CAD build for the part. Positions are in the model's coordinates, mm. Face numbers are marked on the shaded views. A direction names the side the tool comes from. Coordinates: 2 decimals unless noted, no trailing zeros. Write each loop counter-clockwise with the first axis right and the second up, starting at its lowest first coordinate (ties: lowest second). Pieces come first, ordered by that corner, then holes. Notation, with made-up numbers: (17.5, -35) -> (54.5, -35) arc R7 ccw to (54.5, -26) -> close; hole circle Ø10 at (65, 56). An arc over 180 degrees is marked (long way). Answer as CSV lines item,"result".
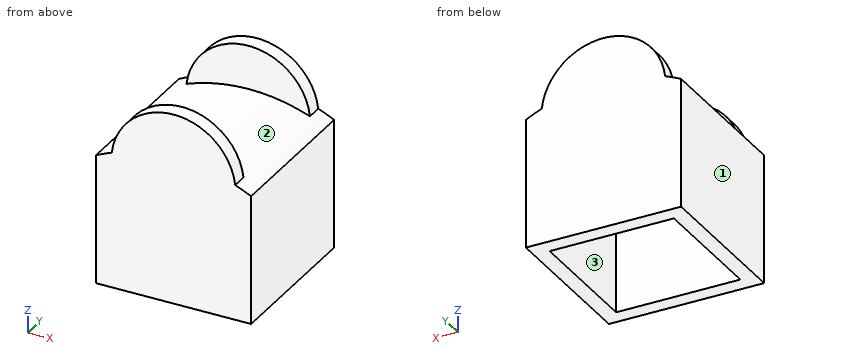
```python
from build123d import *

# Parameters (mm, degrees)
F0_W          = 30
F0_H          = 30
F0_W_2        = 24
F0_H_2        = 24
F1_DEPTH      = 25
F3_DEPTH      = 15
F3_DEPTH_BACK = 15
F5_DEPTH      = 3
F7_DEPTH      = 3


with BuildPart() as f1:
    # F0 (on Top) → F1 (new body)
    with BuildSketch(Plane.XY):
        Rectangle(F0_W, F0_H)
        Rectangle(F0_W_2, F0_H_2, mode=Mode.SUBTRACT)
    extrude(amount=F1_DEPTH)

    # F2 (on Front) → F3 (join, two sides)
    with BuildSketch(Plane.XZ) as f3_sk:
        with BuildLine():
            Line((12, 25), (15, 25))
            ThreePointArc((15, 25), (0, 28.5410196625), (-15, 25))
            Line((-15, 25), (-12, 25))
            ThreePointArc((-12, 25), (0, 27.3109888428), (12, 25))
        make_face()
    extrude(amount=F3_DEPTH)
    extrude(f3_sk.sketch, amount=-F3_DEPTH_BACK)

    # F4 (on face) → F5 (join, through all)
    with BuildSketch(Plane(origin=(0, 15, 0), x_dir=(-1, 0, 0), z_dir=(0, 1, 0))):
        with BuildLine():
            Line((-12, 25), (12, 25))
            ThreePointArc((12, 25), (0, 37), (-12, 25))
        make_face()
    extrude(amount=-F5_DEPTH)

    # F6 (on face) → F7 (join, through all)
    with BuildSketch(Plane.XZ.offset(15)):
        with BuildLine():
            Line((-12, 25), (12, 25))
            ThreePointArc((12, 25), (0, 37), (-12, 25))
        make_face()
    extrude(amount=-F7_DEPTH)


solid = f1.part
```
Item 1: Saw through at C-C on x = -10. Give the cut face in (y, z), and give its area (3 significant figures).
Answer below:
outline,"(-15, 0) -> (-12, 0) -> (-12, 25.72) -> (12, 25.72) -> (12, 0) -> (15, 0) -> (15, 31.63) -> (12, 31.63) -> (12, 27.02) -> (-12, 27.02) -> (-12, 31.63) -> (-15, 31.63) -> close"
area,"221 mm2"
Item 2: Saw through at D-D on x = 1.75. Give the cut face in (y, z).
Answer below:
outline,"(-15, 0) -> (-12, 0) -> (-12, 27.26) -> (12, 27.26) -> (12, 0) -> (15, 0) -> (15, 36.87) -> (12, 36.87) -> (12, 28.5) -> (-12, 28.5) -> (-12, 36.87) -> (-15, 36.87) -> close"
Item 3: Saw through at A-A on z = 16.5. Give the cut face in (x, y), and give its area (3 significant figures).
Answer below:
outline,"(-15, -15) -> (15, -15) -> (15, 15) -> (-15, 15) -> close; hole (-12, -12) -> (12, -12) -> (12, 12) -> (-12, 12) -> close"
area,"324 mm2"
Item 4: Wall check: line 1 (X direction, y = -6.25, z = 14); line 2 (Z direction, x = -0.25, y = -9). Give the ranges that are in metal, low to high. Write a range as from..to.
Answer below:
line 1,"x = -15..-12, 12..15"
line 2,"z = 27.31..28.54"
Item 5: Saw through at B-B on y = -3.25. Give the cut face in (x, z), and give its area (3 significant figures).
Answer below:
outline,"(-15, 0) -> (-12, 0) -> (-12, 25) arc R32.31 cw to (12, 25) -> (12, 0) -> (15, 0) -> (15, 25) arc R33.54 ccw to (-15, 25) -> close"
area,"184 mm2"
Item 6: 3-axis set-ups, long thin cutter, end or side, ignore diameter. For the marked faces 1, 2 and 3: which of +Z, -Z, +X, -X, +Y, -Y reach the whole face in a straight line?
Answer below:
face 1,"+Z, -Z, -X, +Y, -Y"
face 2,"+Z"
face 3,"-Z"
